For this review, take the finished solid that the model builds, in its own axes (mm). A direction names the side the tool comes from. Give positions to 0.01 mm unless a question says otherwise; leave off trailing zeros. Loops run counter-clockwise (first coordinate to the right, second up) from the corner with the lowest first, then second, coordinate; pieces in that order, holes last. Notation, with made-up numbers: M 46,66 L 60,66 A15 ccw 60,82 Z; hole C 59.5,3 d8. An arc over 180 degrees is marked long. Use CSV: the item, a comma, the result in double quotes. Start each with the question number.
1. Take a section at C-C, the plane z = -11. Write out the cut boundary in (x, y).
2. Take a section at D-D, the plane y = 32.5. Write out the cut boundary in (x, z), and give its area (3 significant figures).
3. The part is to be moulded in two halves that separate along X. For faces 5 (the face through (-1, 59, 31)), 6 (the face through (-37.5, 30, 0)), 7 (the face through (82.5, 77, -8)), say which applies: pulls with the +X half, pulls with the -X half, needs draft (parallel to the pull), parting line crosses it, or undercut.
4. Take a section at A-A, the plane y = 78.75. Write out the cut boundary in (x, z).
5. To check wall thickness, follow line 1 (Z direction, x = -79.3, y = 67.75); line 2 (Z direction, x = -2, y = 74); line 3 (X direction, y = 12, z = -29). State the ranges of each line that lie inside material, in increasing order. Write a range as [from, to].
6. Insertion check: P1, Ø4, axis at x = 65, z = 26, coming from the -Y side; P2, Ø8.5, axis at y = 76, z = 4, coming from the +X side; P3, Ø5, axis at x = 2.5, z = -22, coming from the +Y side; P4, Ø4, axis at y = 20, z = -1, coming from the -X side. Each pin has a flat end and moves straight along its axis. Give the tip position at first contact, or say it passes through.
7. Tool access review of faces 1 (the face through (-60, 60, 0)), 2 (the face through (-33.5, 32, 0)), 3 (the face through (37.5, 30, 0)), 4 (the face through (-1, 56, 35)): name each direction out of +Z, -Z, +X, -X, +Y, -Y from which nothing blocks a thin tool from reaching the whole face with its end or side.
8. Take a section at B-B, the plane x = -5. Write out the cut boundary in (y, z).
from build123d import *

# Parameters (mm, degrees)
SKETCH1_W                = 75
SKETCH1_H                = 40
SKETCH1_R                = 5
SKETCH1_R_2              = 1.7
SKETCH1_R_3              = 1.197563381
SKETCH1_W_2              = 5
SKETCH1_H_2              = 20
BOSS_EXTRUDE1_DEPTH      = 3
CUT_EXTRUDE1_DEPTH       = 43.605750786
CUT_EXTRUDE1_DEPTH_BACK  = 43.605750786
SKETCH2_W                = 67
SKETCH2_H                = 28
BOSS_EXTRUDE3_DEPTH      = 90
BOSS_EXTRUDE3_DEPTH_BACK = 3
SKETCH6_W                = 67
SKETCH6_H                = 11
CUT_EXTRUDE4_DEPTH       = 104.591746776
SKETCH7_W                = 70
SKETCH7_H                = 37
BOSS_EXTRUDE4_DEPTH      = 45
SKETCH8_W                = 45
SKETCH8_H                = 62
CUT_EXTRUDE6_DEPTH       = 29
SKETCH9_R                = 1.25
SKETCH9_R_2              = 10.5
CUT_EXTRUDE8_DEPTH       = 193.611006954
SKETCH11_W               = 45
SKETCH11_H               = 4
CUT_EXTRUDE9_DEPTH       = 143.671826231


with BuildPart() as part:
    # Sketch1 → Boss-Extrude1 (new body)
    with BuildSketch(Plane(origin=(0, 0, 0), x_dir=(1, 0, 0), z_dir=(0, 1, 0))):
        Rectangle(SKETCH1_W, SKETCH1_H)
        with Locations(Location((-21, 0, 0), (0, 0, 270))):
            Circle(SKETCH1_R, mode=Mode.SUBTRACT)
        with Locations(Location((-30, 8.25, 0), (0, 0, 270))):
            Circle(SKETCH1_R_2, mode=Mode.SUBTRACT)
        with Locations(Location((-12, 8.25, 0), (0, 0, 270))):
            Circle(SKETCH1_R_2, mode=Mode.SUBTRACT)
        with Locations(Location((-12, -8.25, 0), (0, 0, 270))):
            Circle(SKETCH1_R_2, mode=Mode.SUBTRACT)
        with Locations(Location((-30, -8.25, 0), (0, 0, 270))):
            Circle(SKETCH1_R_2, mode=Mode.SUBTRACT)
        with Locations(Location((12, 8.25, 0), (0, 0, 90))):
            Circle(SKETCH1_R_2, mode=Mode.SUBTRACT)
        with Locations(Location((12, -8.25, 0), (0, 0, 90))):
            Circle(SKETCH1_R_2, mode=Mode.SUBTRACT)
        with Locations(Location((21, 0, 0), (0, 0, 90))):
            Circle(SKETCH1_R, mode=Mode.SUBTRACT)
        with Locations(Location((30, -8.25, 0), (0, 0, 90))):
            Circle(SKETCH1_R_2, mode=Mode.SUBTRACT)
        with Locations(Location((30, 8.25, 0), (0, 0, 90))):
            Circle(SKETCH1_R_2, mode=Mode.SUBTRACT)
        with Locations(Location((-30, -17.5, 0), (0, 0, 270))):
            Circle(SKETCH1_R_3, mode=Mode.SUBTRACT)
        with Locations(Location((-12, -17.5, 0), (0, 0, 270))):
            Circle(SKETCH1_R_3, mode=Mode.SUBTRACT)
        with Locations(Location((12, -17.5, 0), (0, 0, 90))):
            Circle(SKETCH1_R_3, mode=Mode.SUBTRACT)
        with Locations(Location((30, -17.5, 0), (0, 0, 90))):
            Circle(SKETCH1_R_3, mode=Mode.SUBTRACT)
        with Locations(Location((30, 17.5, 0), (0, 0, 270))):
            Circle(SKETCH1_R_3, mode=Mode.SUBTRACT)
        with Locations(Location((12, 17.5, 0), (0, 0, 270))):
            Circle(SKETCH1_R_3, mode=Mode.SUBTRACT)
        with Locations(Location((-12, 17.5, 0), (0, 0, 90))):
            Circle(SKETCH1_R_3, mode=Mode.SUBTRACT)
        with Locations(Location((-30, 17.5, 0), (0, 0, 90))):
            Circle(SKETCH1_R_3, mode=Mode.SUBTRACT)
        Rectangle(SKETCH1_W_2, SKETCH1_H_2, mode=Mode.SUBTRACT)
    extrude(amount=BOSS_EXTRUDE1_DEPTH)

    # Sketch2 → Cut-Extrude1 (cut, two sides: drawn at the far end of the back side and taken through both)
    with BuildSketch(Plane(origin=(0, 3, 0), x_dir=(1, 0, 0), z_dir=(0, 1, 0)).offset(-CUT_EXTRUDE1_DEPTH_BACK)):
        Rectangle(SKETCH2_W, SKETCH2_H)
    extrude(amount=CUT_EXTRUDE1_DEPTH + CUT_EXTRUDE1_DEPTH_BACK, mode=Mode.SUBTRACT)

    # Sketch3 → Boss-Extrude3 (add, two sides: drawn at the far end of the back side and taken through both)
    with BuildSketch(Plane(origin=(0, 3, 0), x_dir=(1, 0, 0), z_dir=(0, 1, 0)).offset(-BOSS_EXTRUDE3_DEPTH_BACK)):
        Polygon((37.5, -35), (37.5, -20), (33.5, -20), (-33.5, -20), (-37.5, -20), (-37.5, -35), align=None)
        Polygon((33.5, 20), (37.5, 20), (37.5, 35), (-37.5, 35), (-37.5, 20), (-33.5, 20), align=None)
        Polygon((37.5, -20), (37.5, 20), (33.5, 20), (33.5, 14), (33.5, -14), (33.5, -20), align=None)
        Polygon((-33.5, 14), (-33.5, 20), (-37.5, 20), (-37.5, -20), (-33.5, -20), (-33.5, -14), align=None)
    extrude(amount=BOSS_EXTRUDE3_DEPTH + BOSS_EXTRUDE3_DEPTH_BACK)

    # Sketch6 → Cut-Extrude4 (cut, through all)
    with BuildSketch(Plane(origin=(0, 3, 0), x_dir=(1, 0, 0), z_dir=(0, 1, 0))):
        with Locations((0, -25.5)):
            Rectangle(SKETCH6_W, SKETCH6_H)
        with Locations((0, 25.5)):
            Rectangle(SKETCH6_W, SKETCH6_H)
    extrude(amount=CUT_EXTRUDE4_DEPTH, mode=Mode.SUBTRACT)

    # Sketch7 → Boss-Extrude4 (add)
    with BuildSketch(Plane.ZY.offset(37.5)):
        with Locations((0, 74.5)):
            Rectangle(SKETCH7_W, SKETCH7_H)
    boss_extrude4 = extrude(amount=BOSS_EXTRUDE4_DEPTH)

    # Mirror2: Boss-Extrude4 across plane
    add(boss_extrude4.mirror(Plane(origin=(0, 0, 0), x_dir=(0, 0, 1), z_dir=(1, 0, 0))))

    # Sketch8 → Cut-Extrude6 (cut)
    with BuildSketch(Plane(origin=(0, 93, 0), x_dir=(1, 0, 0), z_dir=(0, 1, 0))):
        with Locations((-56, 0)):
            Rectangle(SKETCH8_W, SKETCH8_H)
        with Locations((56, 0)):
            Rectangle(SKETCH8_W, SKETCH8_H)
    extrude(amount=-CUT_EXTRUDE6_DEPTH, mode=Mode.SUBTRACT)

    # Sketch9 → Cut-Extrude8 (cut, through all)
    with BuildSketch(Plane.ZY.offset(82.5)):
        with Locations((-27.75, 89.75)):
            Circle(SKETCH9_R)
        with Locations((-27.75, 67.75)):
            Circle(SKETCH9_R)
        with Locations((4.25, 78.75)):
            Circle(SKETCH9_R_2)
        with Locations((12.25, 67.75)):
            Circle(SKETCH9_R)
        with Locations((12.25, 89.75)):
            Circle(SKETCH9_R)
    extrude(amount=-CUT_EXTRUDE8_DEPTH, mode=Mode.SUBTRACT)

    # Sketch11 → Cut-Extrude9 (cut, through all)
    with BuildSketch(Plane.XY.offset(35)):
        with Locations((-60, 58)):
            Rectangle(SKETCH11_W, SKETCH11_H)
        with Locations((60, 58)):
            Rectangle(SKETCH11_W, SKETCH11_H)
    extrude(amount=-CUT_EXTRUDE9_DEPTH, mode=Mode.SUBTRACT)


solid = part.part
Result set:
1,outline,"M -82.5,60 L -37.5,60 L -37.5,0 L -33.5,0 L -33.5,64 L -78.5,64 L -78.5,93 L -82.5,93 Z; M 33.5,0 L 37.5,0 L 37.5,60 L 82.5,60 L 82.5,93 L 78.5,93 L 78.5,64 L 33.5,64 Z"
2,outline,"M -37.5,-35 L 37.5,-35 L 37.5,35 L -37.5,35 Z; hole M -33.5,-31 L 33.5,-31 L 33.5,31 L -33.5,31 Z"
2,area,"1,100 mm2"
3,face 5,"undercut"
3,face 6,"pulls with the -X half"
3,face 7,"pulls with the +X half"
4,outline,"M -82.5,-35 L 82.5,-35 L 82.5,-6.25 L 78.5,-6.25 L 78.5,-31 L -78.5,-31 L -78.5,-6.25 L -82.5,-6.25 Z; M -82.5,14.75 L -78.5,14.75 L -78.5,31 L 78.5,31 L 78.5,14.75 L 82.5,14.75 L 82.5,35 L -82.5,35 Z"
5,line 1,"[-35, -29], [-26.5, 11], [13.5, 35]"
5,line 2,"[-35, -31], [31, 35]"
5,line 3,"[-37.5, -33.5], [33.5, 37.5]"
6,P1,"y = 60"
6,P2,"through"
6,P3,"y = 3"
6,P4,"x = -37.5"
7,face 1,"+Z, -Z, -X, -Y"
7,face 2,"+Y"
7,face 3,"+Z, -Z, +X, -Y"
7,face 4,"+Z, +X, -X, +Y, -Y"
8,outline,"M 0,-35 L 93,-35 L 93,-31 L 3,-31 L 3,-14 L 0,-14 Z; M 0,14 L 3,14 L 3,31 L 93,31 L 93,35 L 0,35 Z"
